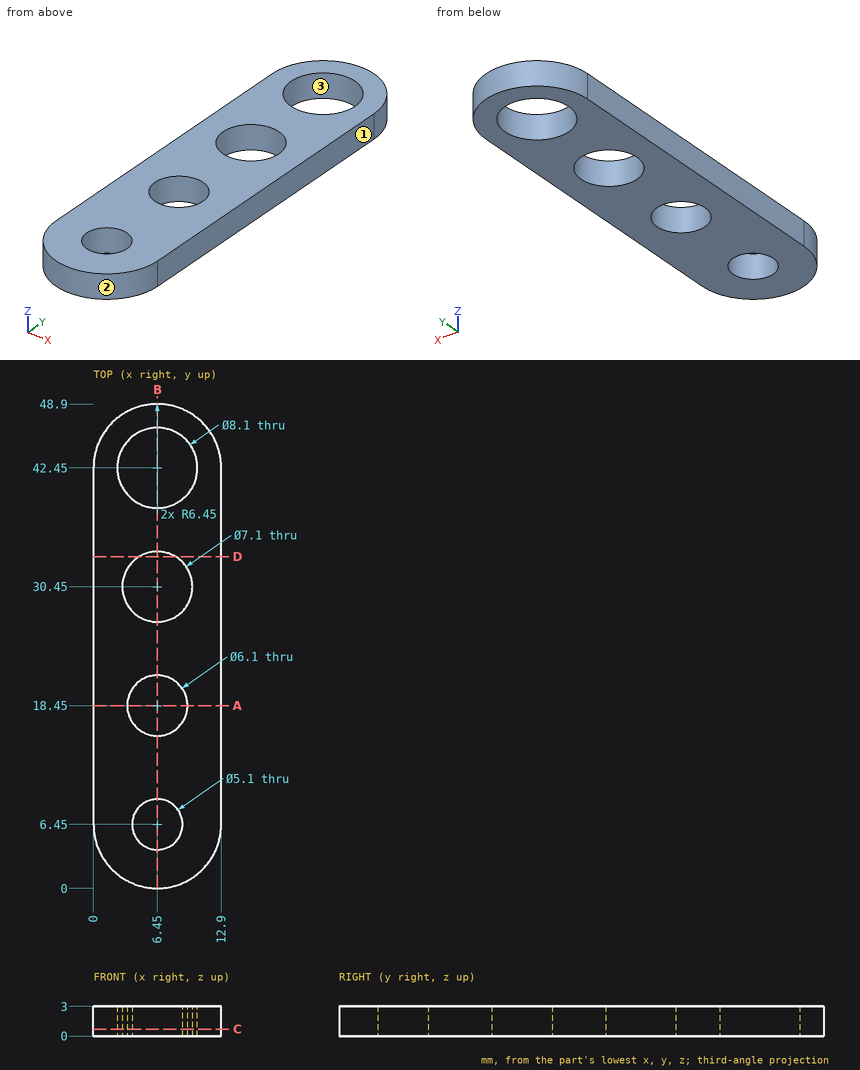
Drawing for the job (mm, zero at the part's lowest x, y, z). Round coordinates to 2 decimals unless told otherwise and drop trailing zeros. Loops run counter-clockwise (first coordinate to the right, second up) from the corner with the lowest first, then second, coordinate; pieces in that order, holes last. Notation, with made-up numbers: (-21, 17) -> (2, 17) arc R13 ccw to (2, 26) -> close; hole circle Ø10 at (65, 56.5). An arc over 180 degrees is marked (long way). Answer as CSV lines item,"result". Start each with the question number.
1) Probe line 1 along Y through (x, z) = (6.45, 0.75); line 2 along Y through (x, z) = (5, 1.8); line 3 along Y through (x, z) = (9.25, 1.3). List the from-to ranges inside material, lowest first.
2) Slice it at D-D (y = 33.5). List the corners of the cut face in (x, z), plus the area to 3 significant figures.
3) Slice it at A-A (y = 18.45). List the corners of the cut face in (x, z).
4) Slice it at C-C (z = 0.7). List the corners of the cut face in (x, y), plus the area to 3 significant figures.
5) Pin check, flat tips, straight feed: P1, Ø1.5, axis at x = 2.5, z = 2, coming from the +Y side; P2, Ø1.5, axis at x = 10, z = 1, coming from the -Y side. Stop position of each tip, or through.
6) Slice it at B-B (x = 6.45). List the corners of the cut face in (y, z).
7) Mould opens along X. For the marked faces 1, 2 and 3 say: +X half, -X half, draft (parallel to the pull), parting line (faces both ways), or undercut.
Filled in:
1,line 1,"y = 0 to 3.9, 9 to 15.4, 21.5 to 26.9, 34 to 38.4, 46.5 to 48.9"
1,line 2,"y = 0.17 to 4.35, 8.55 to 15.77, 21.13 to 27.21, 33.69 to 38.67, 46.23 to 48.73"
1,line 3,"y = 0.64 to 17.24, 19.66 to 28.27, 32.63 to 39.52, 45.38 to 48.26"
2,outline,"(0, 0) -> (4.63, 0) -> (4.63, 3) -> (0, 3) -> close; (8.27, 0) -> (12.9, 0) -> (12.9, 3) -> (8.27, 3) -> close"
2,area,"27.8 mm2"
3,outline,"(0, 0) -> (3.4, 0) -> (3.4, 3) -> (0, 3) -> close; (9.5, 0) -> (12.9, 0) -> (12.9, 3) -> (9.5, 3) -> close"
4,outline,"(0, 6.45) arc R6.45 ccw to (12.9, 6.45) -> (12.9, 42.45) arc R6.45 ccw to (0, 42.45) -> close; hole circle Ø8.1 at (6.45, 42.45); hole circle Ø7.1 at (6.45, 30.45); hole circle Ø6.1 at (6.45, 18.45); hole circle Ø5.1 at (6.45, 6.45)"
4,area,"454 mm2"
5,P1,"stops at y = 48.05"
5,P2,"stops at y = 0.64"
6,outline,"(0, 0) -> (3.9, 0) -> (3.9, 3) -> (0, 3) -> close; (9, 0) -> (15.4, 0) -> (15.4, 3) -> (9, 3) -> close; (21.5, 0) -> (26.9, 0) -> (26.9, 3) -> (21.5, 3) -> close; (34, 0) -> (38.4, 0) -> (38.4, 3) -> (34, 3) -> close; (46.5, 0) -> (48.9, 0) -> (48.9, 3) -> (46.5, 3) -> close"
7,face 1,"+X half"
7,face 2,"parting line"
7,face 3,"undercut"
